Work out the finished part from the listing and answer in its coordinate system (mm). Give positions to 0.01 mm unless a question says otherwise; leave off trailing zeros. Order: outer loops, then holes, each group sorted by start corner. A loop starts at its lowest first (then second) coordinate and runs counter-clockwise, first axis right, second up. Notation, with made-up numbers: (-38.75, -17) - (-2.75, -17) arc R6 ccw to (-2.75, -6) - close; hole circle Ø5 at (63, 82). An arc over 180 degrees is marked (long way). Put each result on its own line as item: value.
```python
from build123d import *

# Parameters (mm, degrees)
SKETCH_W        = 50
SKETCH_H        = 92
SKETCH_R        = 2.625
SKETCH_R_2      = 1.625
SKETCH_R_3      = 12
PAD_DEPTH       = 6
CHAMFER_SIZE    = 0.5
CHAMFER001_SIZE = 0.25


with BuildPart() as part:
    # Sketch → Pad (new body)
    with BuildSketch(Plane.XY):
        Rectangle(SKETCH_W, SKETCH_H)
        with Locations((-18, 40)):
            Circle(SKETCH_R, mode=Mode.SUBTRACT)
        with Locations((18, 40)):
            Circle(SKETCH_R, mode=Mode.SUBTRACT)
        with Locations((-18, -40)):
            Circle(SKETCH_R, mode=Mode.SUBTRACT)
        with Locations((18, -40)):
            Circle(SKETCH_R, mode=Mode.SUBTRACT)
        with Locations((-15.5, 15.5)):
            Circle(SKETCH_R_2, mode=Mode.SUBTRACT)
        with Locations((15.5, 15.5)):
            Circle(SKETCH_R_2, mode=Mode.SUBTRACT)
        with Locations((-15.5, -15.5)):
            Circle(SKETCH_R_2, mode=Mode.SUBTRACT)
        with Locations((15.5, -15.5)):
            Circle(SKETCH_R_2, mode=Mode.SUBTRACT)
        Circle(SKETCH_R_3, mode=Mode.SUBTRACT)
    extrude(amount=PAD_DEPTH)

    # Chamfer
    chamfer_edges = [part.edges().sort_by_distance(p)[0] for p in [
        (-12, 0, 6),
        (-12, 0, 0),
    ]]
    chamfer(chamfer_edges, length=CHAMFER_SIZE)

    # Chamfer001
    chamfer001_edges = [part.edges().sort_by_distance(p)[0] for p in [
        (-17.125, 15.5, 6),
        (-17.125, -15.5, 6),
        (13.875, -15.5, 6),
        (13.875, 15.5, 6),
        (13.875, -15.5, 0),
        (13.875, 15.5, 0),
        (-17.125, -15.5, 0),
        (-17.125, 15.5, 0),
    ]]
    chamfer(chamfer001_edges, length=CHAMFER001_SIZE)


solid = part.part
```
(1) Given pin 1 (3.5 mm diameter, centred on x = -15.5, y = -15.5, fed in from -Z) (3 decimals), flat-ended and moving along its own axis, determine where the tip first touches the part or whether it passes through.
Geometry check:
pin 1: stops at z = 0.125
(2) Straight lines are drawn through the part: line 1 (Y direction, x = 18, z = 1.95) (3 decimals); line 2 (Y direction, x = -15, z = 0.4); line 3 (Y direction, x = 0.5, z = 1.85). For each, find the intervals that lie inside material, in ascending order.
Geometry check:
line 1: y = -46 to -42.625, -37.375 to 37.375, 42.625 to 46
line 2: y = -46 to -17.05, -13.95 to 13.95, 17.05 to 46
line 3: y = -46 to -11.99, 11.99 to 46
(3) Determine the mould class of faces 1 (the face through (-11.99, 0.53, 2.96)), 2 (the face through (0, -46, 3)), 3 (the face through (0, 46, 3)), 4 (the face through (-25, -1, 3)) for opening direction Y: pulls with the +Y half, pulls with the -Y half, needs draft (parallel to the pull), parting line crosses it, or undercut.
Geometry check:
face 1: undercut
face 2: pulls with the -Y half
face 3: pulls with the +Y half
face 4: needs draft
(4) Section B-B, the plane x = 0 is taken. Write down the section's boundary in (y, z).
Geometry check:
outline: (-46, 0) - (-12.5, 0) - (-12, 0.5) - (-12, 5.5) - (-12.5, 6) - (-46, 6) - close; (12, 0.5) - (12.5, 0) - (46, 0) - (46, 6) - (12.5, 6) - (12, 5.5) - close
(5) Section A-A, the plane y = 15.5 is taken. Write down the section's boundary in (x, z) (3 decimals), then the cut area to 3 significant figures.
Geometry check:
outline: (-25, 0) - (-17.375, 0) - (-17.125, 0.25) - (-17.125, 5.75) - (-17.375, 6) - (-25, 6) - close; (-13.875, 0.25) - (-13.625, 0) - (13.625, 0) - (13.875, 0.25) - (13.875, 5.75) - (13.625, 6) - (-13.625, 6) - (-13.875, 5.75) - close; (17.125, 0.25) - (17.375, 0) - (25, 0) - (25, 6) - (17.375, 6) - (17.125, 5.75) - close
area: 261 mm²
(6) Section C-C, the plane y = -40 is taken. Write down the section's boundary in (x, z) (3 decimals), then the cut area to 3 significant figures.
Geometry check:
outline: (-25, 0) - (-20.625, 0) - (-20.625, 6) - (-25, 6) - close; (-15.375, 0) - (15.375, 0) - (15.375, 6) - (-15.375, 6) - close; (20.625, 0) - (25, 0) - (25, 6) - (20.625, 6) - close
area: 237 mm²
(7) Section D-D, the plane y = 39 is taken. Write down the section's boundary in (x, z), then the cut area to 3 significant figures.
Geometry check:
outline: (-25, 0) - (-20.43, 0) - (-20.43, 6) - (-25, 6) - close; (-15.57, 0) - (15.57, 0) - (15.57, 6) - (-15.57, 6) - close; (20.43, 0) - (25, 0) - (25, 6) - (20.43, 6) - close
area: 242 mm²
